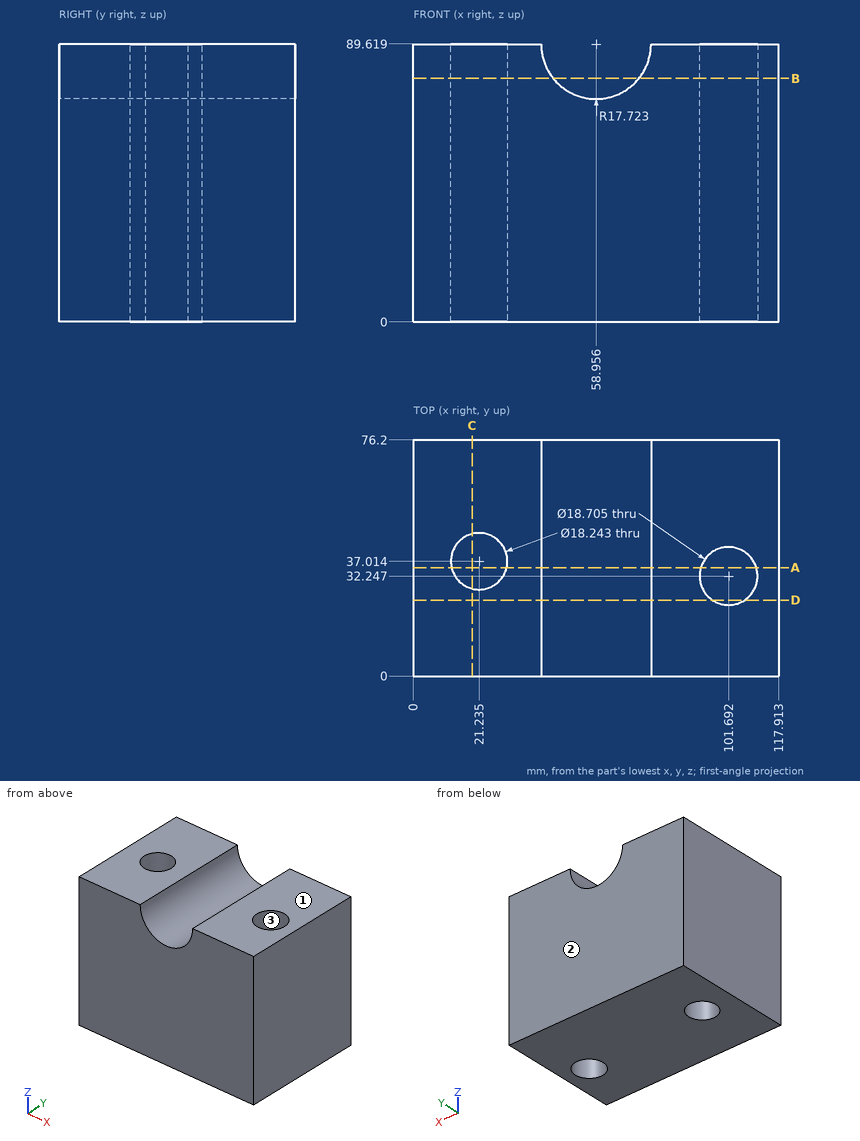
Design review of the part shown in the three views and the two pictorial views. Dimensions are in mm from the part's minimum x, y and z. Round coordinates to 2 decimals unless told otherwise and drop trailing zeros. Write each loop counter-clockwise with the first axis right and the second up, starting at its lowest first coordinate (ties: lowest second). Pieces come first, ordered by that corner, then holes.
Item 1: For pin 1 Ø1.5 at (x, z) = (32, 56.5) entering from -Y; pin 2 Ø14.5 at (x, y) = (21.23, 37.01) entering from +Z; pin 3 Ø10 at (x, y) = (56.5, 23) entering from +Z, all flat-tipped, find the tip position at first contact; note any pin that passes through.
Item 2: Draft analysis for pull direction Y (two halves, no side actions). For the marked faces 1, 2 and 3, state which applies: released by +Y, released by -Y, zero draft, split by the parting line, or undercut.
Item 3: Consider section D-D on y = 24.5. Give the boundary of the cut face in (x, z) (1 decimal).
Item 4: Wall thickness on L1, parallel to X at y = 35.5, z = 64; L2, parallel to X at y = 31, z = 42 (1 decimal); L3, parallel to Y at x = 94, z = 10 (1 decimal): over which ranges is each line inside the solid? List them lowest first.
Item 5: Consider section A-A on y = 35. Give the boundary of the cut face in (x, z) (1 decimal).
Item 6: Consider section B-B on z = 78.5. Give the boundary of the cut face in (x, y) (1 decimal).
Item 7: Consider section C-C on x = 19. Give the boundary of the cut face in (y, z).
Check values:
1. pin 1: stops at y = 0
1. pin 2: passes through
1. pin 3: stops at z = 73.54
2. face 1: zero draft
2. face 2: released by +Y
2. face 3: undercut
3. outline: (0, 0) - (96.5, 0) - (96.5, 89.6) - (76.7, 89.6) arc R17.7 cw to (41.2, 89.6) - (0, 89.6) - close; (106.9, 0) - (117.9, 0) - (117.9, 89.6) - (106.9, 89.6) - close
4. L1: x = 0 to 12.24, 30.23 to 92.92, 110.46 to 117.91
4. L2: x = 0 to 14.4, 28.1 to 92.4, 111 to 117.9
4. L3: y = 0 to 26.9, 37.6 to 76.2
5. outline: (0, 0) - (12.3, 0) - (12.3, 89.6) - (0, 89.6) - close; (30.1, 0) - (92.8, 0) - (92.8, 89.6) - (76.7, 89.6) arc R17.7 cw to (41.2, 89.6) - (30.1, 89.6) - close; (110.6, 0) - (117.9, 0) - (117.9, 89.6) - (110.6, 89.6) - close
6. outline: (0, 0) - (45.2, 0) - (45.2, 76.2) - (0, 76.2) - close; (72.8, 0) - (117.9, 0) - (117.9, 76.2) - (72.8, 76.2) - close; hole circle Ø18.2 at (21.2, 37); hole circle Ø18.7 at (101.7, 32.2)
7. outline: (0, 0) - (28.17, 0) - (28.17, 89.62) - (0, 89.62) - close; (45.86, 0) - (76.2, 0) - (76.2, 89.62) - (45.86, 89.62) - close
